The listing builds one solid part. Answer for the finished solid, in the listing's coordinates (mm). A direction names the side the tool comes from. Give positions to 0.01 mm unless a question says otherwise; leave off trailing zeros. Loops run counter-clockwise (first coordinate to the right, second up) from the corner with the lowest first, then second, coordinate; pieces in that order, holes last. Notation, with made-up numbers: (-2, -37) - (19, -37) arc R19 ccw to (19, -23) - close; hole circle Ø2 at (68, 64). An arc over 180 degrees is marked (long way). Write item = value, one per line. Start each with the question number.
1) The part is cut by section D-D on z = -28. Write down the section's boundary in (x, y).
2) Which of the six approach directions +Z, -Z, +X, -X, +Y, -Y give full straight-line access (tool end or side, diameter ignored) to faces 4 (the flat face through (-25, 0, 16)), 5 (the flat face through (-51.657, -16, 16)), 6 (the cylindrical face through (71.625, 4.859, -19.627))?
3) Consider probe 1 along Z at (x, y) = (46.5, -50); probe 2 along X at (y, z) = (12.5, 14); probe 3 along X at (y, z) = (-55, 23.5). Determine where each line is inside the solid, lowest interval first.
4) The part is cut by section B-B on x = 61.5. Write down the section's boundary in (y, z).
5) The part is cut by section C-C on y = -43.5. Write down the section's boundary in (x, z), plus the area to 3 significant figures.
6) Flat-ended cylindrical pins translate along their axes: P1, Ø12, axis at x = -19.5, z = -8, coming from the -Y side (3 decimals); P2, Ø5, axis at y = -12.5, z = -26, coming from the +X side; P3, Ø10, axis at x = -30, z = 14, coming from the +Y side; P4, Ø1.5, axis at x = 47.5, z = -14, coming from the +Y side. Find the tip coordinate at first contact, or state that the pin passes through.
7) The mould has two halves that part along Z. Classify faces 1 (the flat face through (54, -15, 33.351)), 2 (the flat face through (54, -27, 0)), 3 (the flat face through (0, 19, 16)): +Z half, -Z half, draft (parallel to the pull), parting line (faces both ways), or undercut.
8) The part is cut by section A-A on z = 21. Write down the section's boundary in (x, y).
from build123d import *

# Parameters (mm, degrees)
F1_DEPTH = 33.3509109914
F2_R     = 16.1774889393
F3_DEPTH = 39.8117862642


# Not quite as in the source:
# - a feature names something its author has since deleted; it is built from what else it names


with BuildPart() as f1:
    # F0 (on Top) → F1 (new body)
    with BuildSketch(Plane.XY):
        Polygon((75.3069221973, -69.7055906057), (156.8375527859, -13.2772475481), (160.0531488657, 9.1281235218), (163.2687449455, 31.5334945917), (0, 38.3795797825), (0, 0), (-51.6568571329, 0), (-51.6568571329, -32.155841589), (-11.8250846863, -69.7055906057), align=None)
    extrude(amount=F1_DEPTH)

    # F2 (on Top) → F3 (join)
    with BuildSketch(Plane.XY):
        with Locations((56.1946332455, 0)):
            Circle(F2_R)
    extrude(amount=-F3_DEPTH)


solid = f1.part
Answer below:
q1.outline = circle Ø32.35 at (56.19, 0)
q2.face_4 = +Z, -Z, -X, +Y
q2.face_5 = +Z, -Z, -X, +Y, -Y
q2.face_6 = -Z
q3.probe_1 = 0 to 33.35
q3.probe_2 = 0 to 160.54
q3.probe_3 = -27.42 to 96.55
q4.outline = (-69.71, 0) - (-15.28, 0) - (-15.28, -39.81) - (15.28, -39.81) - (15.28, 0) - (35.8, 0) - (35.8, 33.35) - (-69.71, 33.35) - close
q5.outline = (-39.62, 0) - (113.17, 0) - (113.17, 33.35) - (-39.62, 33.35) - close
q5.area = 5,100 mm2
q6.P1 = through
q6.P2 = 68.91
q6.P3 = 0
q6.P4 = 14.09
q7.face_1 = +Z half
q7.face_2 = -Z half
q7.face_3 = draft
q8.outline = (-51.66, -32.16) - (-11.83, -69.71) - (75.31, -69.71) - (156.84, -13.28) - (163.27, 31.53) - (0, 38.38) - (0, 0) - (-51.66, 0) - close
